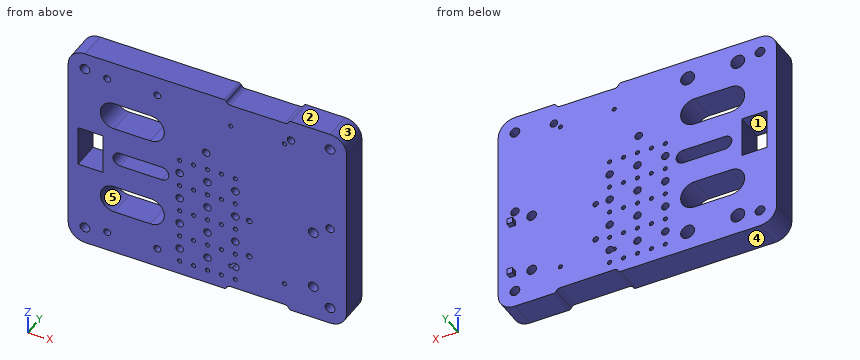
```python
from build123d import *

# Parameters (mm, degrees)
SKETCH_1_W          = 100
SKETCH_1_H          = 75
SKETCH_1_R          = 1.75
SKETCH_1_R_2        = 1.25
SKETCH_1_R_3        = 0.75
SKETCH_1_R_4        = 1.5
SKETCH_1_W_2        = 9
SKETCH_1_H_2        = 14.5
EXTRUDE_1_DEPTH     = 10
FILLET_5_R          = 6
CUT_EXTRUDE_1_REACH = 12
SKETCH_2_R          = 1.35
SKETCH_2_R_2        = 1.75
SKETCH_2_R_3        = 1
SKETCH_3_R          = 2.5
CUT_EXTRUDE_2_DEPTH = 7
SKETCH_4_W          = 2
SKETCH_4_H          = 2
EXTRUDE_2_DEPTH     = 2
CUT_EXTRUDE_3_DEPTH = 36.8
FILLET_6_R          = 1
SKETCH_6_R          = 1.35
SKETCH_6_R_2        = 0.75
CUT_EXTRUDE_4_DEPTH = 36.8


with BuildPart() as part:
    # Эскиз1 → Бобышка-Вытянуть1 (new body)
    with BuildSketch(Plane(origin=(0, 0, 0), x_dir=(1, 0, 0), z_dir=(0, 1, 0))):
        with Locations((50, 37.5)):
            Rectangle(SKETCH_1_W, SKETCH_1_H)
        with Locations((6, 69)):
            Circle(SKETCH_1_R, mode=Mode.SUBTRACT)
        with Locations((94, 69)):
            Circle(SKETCH_1_R, mode=Mode.SUBTRACT)
        with Locations((94, 6)):
            Circle(SKETCH_1_R, mode=Mode.SUBTRACT)
        with Locations((6, 6)):
            Circle(SKETCH_1_R, mode=Mode.SUBTRACT)
        with Locations((14, 68)):
            Circle(SKETCH_1_R_2, mode=Mode.SUBTRACT)
        with Locations((32, 68)):
            Circle(SKETCH_1_R_2, mode=Mode.SUBTRACT)
        with Locations((32, 7)):
            Circle(SKETCH_1_R_2, mode=Mode.SUBTRACT)
        with Locations((14, 7)):
            Circle(SKETCH_1_R_2, mode=Mode.SUBTRACT)
        with Locations((58.35, 65.3)):
            Circle(SKETCH_1_R_3, mode=Mode.SUBTRACT)
        with Locations((77.65, 65.3)):
            Circle(SKETCH_1_R_3, mode=Mode.SUBTRACT)
        with Locations((77.65, 9.7)):
            Circle(SKETCH_1_R_3, mode=Mode.SUBTRACT)
        with Locations((58.35, 9.7)):
            Circle(SKETCH_1_R_3, mode=Mode.SUBTRACT)
        with Locations((94, 37.5)):
            Circle(SKETCH_1_R_4, mode=Mode.SUBTRACT)
        with BuildLine():
            Line((16.5, 59), (29.5, 59))
            ThreePointArc((29.5, 59), (34.5, 54), (29.5, 49))
            Line((29.5, 49), (16.5, 49))
            ThreePointArc((16.5, 49), (11.5, 54), (16.5, 59))
        make_face(mode=Mode.SUBTRACT)
        with BuildLine():
            Line((16.5, 16), (29.5, 16))
            ThreePointArc((29.5, 16), (34.5, 21), (29.5, 26))
            Line((29.5, 26), (16.5, 26))
            ThreePointArc((16.5, 26), (11.5, 21), (16.5, 16))
        make_face(mode=Mode.SUBTRACT)
        with Locations((8, 37.5)):
            Rectangle(SKETCH_1_W_2, SKETCH_1_H_2, mode=Mode.SUBTRACT)
    extrude(amount=EXTRUDE_1_DEPTH)

    # Скругление5
    fillet_5_edges = [part.edges().sort_by_distance(p)[0] for p in [
        (0, 5, -75),
        (100, 5, -75),
        (100, 5, 0),
        (0, 5, 0),
    ]]
    fillet(fillet_5_edges, radius=FILLET_5_R)

    # Эскиз2 → Вырез-Вытянуть1 (cut, up to next)
    with BuildSketch(Plane.XZ, mode=Mode.PRIVATE) as cut_extrude_1_sk1:
        with Locations((80, -7.5)):
            Circle(SKETCH_2_R)
    cut_extrude_1_tool1 = extrude(cut_extrude_1_sk1.sketch, amount=-CUT_EXTRUDE_1_REACH, mode=Mode.PRIVATE) & part.part
    add(cut_extrude_1_tool1.solids().sort_by_distance((80, 0, -7.5))[0], mode=Mode.SUBTRACT)
    # Эскиз2 → Вырез-Вытянуть1 (cut, up to next)
    with BuildSketch(Plane.XZ, mode=Mode.PRIVATE) as cut_extrude_1_sk2:
        with Locations((88, -62.75)):
            Circle(SKETCH_2_R_2)
    cut_extrude_1_tool2 = extrude(cut_extrude_1_sk2.sketch, amount=-CUT_EXTRUDE_1_REACH, mode=Mode.PRIVATE) & part.part
    add(cut_extrude_1_tool2.solids().sort_by_distance((88, 0, -62.75))[0], mode=Mode.SUBTRACT)
    # Эскиз2 → Вырез-Вытянуть1 (cut, up to next)
    with BuildSketch(Plane.XZ, mode=Mode.PRIVATE) as cut_extrude_1_sk3:
        with Locations((88, -41.25)):
            Circle(SKETCH_2_R_2)
    cut_extrude_1_tool3 = extrude(cut_extrude_1_sk3.sketch, amount=-CUT_EXTRUDE_1_REACH, mode=Mode.PRIVATE) & part.part
    add(cut_extrude_1_tool3.solids().sort_by_distance((88, 0, -41.25))[0], mode=Mode.SUBTRACT)
    # Эскиз2 → Вырез-Вытянуть1 (cut, up to next)
    with BuildSketch(Plane.XZ, mode=Mode.PRIVATE) as cut_extrude_1_sk4:
        with Locations((49.550909155, -23.473456754)):
            Circle(SKETCH_2_R)
    cut_extrude_1_tool4 = extrude(cut_extrude_1_sk4.sketch, amount=-CUT_EXTRUDE_1_REACH, mode=Mode.PRIVATE) & part.part
    add(cut_extrude_1_tool4.solids().sort_by_distance((49.550909, 0, -23.473457))[0], mode=Mode.SUBTRACT)
    # Эскиз2 → Вырез-Вытянуть1 (cut, up to next)
    with BuildSketch(Plane.XZ, mode=Mode.PRIVATE) as cut_extrude_1_sk5:
        with Locations((65, -59)):
            Circle(SKETCH_2_R_3)
    cut_extrude_1_tool5 = extrude(cut_extrude_1_sk5.sketch, amount=-CUT_EXTRUDE_1_REACH, mode=Mode.PRIVATE) & part.part
    add(cut_extrude_1_tool5.solids().sort_by_distance((65, 0, -59))[0], mode=Mode.SUBTRACT)
    # Эскиз2 → Вырез-Вытянуть1 (cut, up to next)
    with BuildSketch(Plane.XZ, mode=Mode.PRIVATE) as cut_extrude_1_sk6:
        with Locations((65, -45)):
            Circle(SKETCH_2_R_3)
    cut_extrude_1_tool6 = extrude(cut_extrude_1_sk6.sketch, amount=-CUT_EXTRUDE_1_REACH, mode=Mode.PRIVATE) & part.part
    add(cut_extrude_1_tool6.solids().sort_by_distance((65, 0, -45))[0], mode=Mode.SUBTRACT)
    # Эскиз2 → Вырез-Вытянуть1 (cut, up to next)
    with BuildSketch(Plane.XZ, mode=Mode.PRIVATE) as cut_extrude_1_sk7:
        with BuildLine():
            Line((18.612528652, -35), (33.612528652, -35))
            ThreePointArc((33.612528652, -35), (36.112528652, -37.5), (33.612528652, -40))
            Line((33.612528652, -40), (18.612528652, -40))
            ThreePointArc((18.612528652, -40), (16.112528652, -37.5), (18.612528652, -35))
        make_face()
    cut_extrude_1_tool7 = extrude(cut_extrude_1_sk7.sketch, amount=-CUT_EXTRUDE_1_REACH, mode=Mode.PRIVATE) & part.part
    add(cut_extrude_1_tool7.solids().sort_by_distance((26.112529, 0, -37.5))[0], mode=Mode.SUBTRACT)

    # Эскиз3 → Вырез-Вытянуть2 (cut)
    with BuildSketch(Plane(origin=(0, 10, 0), x_dir=(1, 0, 0), z_dir=(0, 1, 0))):
        with Locations((14, 68)):
            Circle(SKETCH_3_R)
        with Locations((32, 68)):
            Circle(SKETCH_3_R)
        with Locations((14, 7)):
            Circle(SKETCH_3_R)
        with Locations((32, 7)):
            Circle(SKETCH_3_R)
    extrude(amount=-CUT_EXTRUDE_2_DEPTH, mode=Mode.SUBTRACT)

    # Эскиз4 → Бобышка-Вытянуть2 (add)
    with BuildSketch(Plane(origin=(0, 10, 0), x_dir=(1, 0, 0), z_dir=(0, 1, 0))):
        with Locations((94.855745834, 42)):
            Rectangle(SKETCH_4_W, SKETCH_4_H)
        with Locations((94.855745834, 62)):
            Rectangle(SKETCH_4_W, SKETCH_4_H)
    extrude(amount=EXTRUDE_2_DEPTH)

    # Эскиз5 → Вырез-Вытянуть3 (cut)
    with BuildSketch(Plane(origin=(0, 10, 0), x_dir=(1, 0, 0), z_dir=(0, 1, 0))):
        with BuildLine():
            Line((58.204642338, 1.499992816), (77.804642338, 1.439332644))
            ThreePointArc((77.804642338, 1.439332644), (79.299992816, -0.06530251), (77.795357662, -1.560652988))
            Line((77.795357662, -1.560652988), (58.195357662, -1.499992816))
            ThreePointArc((58.195357662, -1.499992816), (56.700007184, 0.004642338), (58.204642338, 1.499992816))
        make_face()
        with BuildLine():
            Line((58.204642338, 73.500007184), (77.804642338, 73.560667356))
            ThreePointArc((77.804642338, 73.560667356), (79.299992816, 75.06530251), (77.795357662, 76.560652988))
            Line((77.795357662, 76.560652988), (58.195357662, 76.499992816))
            ThreePointArc((58.195357662, 76.499992816), (56.700007184, 74.995357662), (58.204642338, 73.500007184))
        make_face()
    extrude(amount=-CUT_EXTRUDE_3_DEPTH, mode=Mode.SUBTRACT)

    # Скругление6
    fillet_6_edges = [part.edges().sort_by_distance(p)[0] for p in [
        (79.298772946, 5, -75),
        (56.7, 5, -75),
        (79.298772946, 5, 0),
        (56.7, 5, 0),
    ]]
    fillet(fillet_6_edges, radius=FILLET_6_R)

    # Эскиз6 → Вырез-Вытянуть4 (cut)
    with BuildSketch(Plane(origin=(0, 10, 0), x_dir=(1, 0, 0), z_dir=(0, 1, 0))):
        with Locations((40, 65)):
            Circle(SKETCH_6_R)
        with Locations((50, 65)):
            Circle(SKETCH_6_R)
        with Locations((60, 65)):
            Circle(SKETCH_6_R)
        with Locations((50, 55)):
            Circle(SKETCH_6_R)
        with Locations((60, 55)):
            Circle(SKETCH_6_R)
        with Locations((50, 45)):
            Circle(SKETCH_6_R)
        with Locations((60, 45)):
            Circle(SKETCH_6_R)
        with Locations((50, 35)):
            Circle(SKETCH_6_R)
        with Locations((60, 35)):
            Circle(SKETCH_6_R)
        with Locations((40, 55)):
            Circle(SKETCH_6_R)
        with Locations((40, 45)):
            Circle(SKETCH_6_R)
        with Locations((40, 35)):
            Circle(SKETCH_6_R)
        with Locations((40, 70)):
            Circle(SKETCH_6_R_2)
        with Locations((45, 70)):
            Circle(SKETCH_6_R_2)
        with Locations((50, 70)):
            Circle(SKETCH_6_R_2)
        with Locations((55, 70)):
            Circle(SKETCH_6_R_2)
        with Locations((60, 70)):
            Circle(SKETCH_6_R_2)
        with Locations((45, 60)):
            Circle(SKETCH_6_R_2)
        with Locations((50, 60)):
            Circle(SKETCH_6_R_2)
        with Locations((55, 60)):
            Circle(SKETCH_6_R_2)
        with Locations((60, 60)):
            Circle(SKETCH_6_R_2)
        with Locations((45, 50)):
            Circle(SKETCH_6_R_2)
        with Locations((50, 50)):
            Circle(SKETCH_6_R_2)
        with Locations((55, 50)):
            Circle(SKETCH_6_R_2)
        with Locations((60, 50)):
            Circle(SKETCH_6_R_2)
        with Locations((45, 40)):
            Circle(SKETCH_6_R_2)
        with Locations((50, 40)):
            Circle(SKETCH_6_R_2)
        with Locations((55, 40)):
            Circle(SKETCH_6_R_2)
        with Locations((60, 40)):
            Circle(SKETCH_6_R_2)
        with Locations((45, 30)):
            Circle(SKETCH_6_R_2)
        with Locations((50, 30)):
            Circle(SKETCH_6_R_2)
        with Locations((55, 30)):
            Circle(SKETCH_6_R_2)
        with Locations((60, 30)):
            Circle(SKETCH_6_R_2)
        with Locations((40, 60)):
            Circle(SKETCH_6_R_2)
        with Locations((40, 50)):
            Circle(SKETCH_6_R_2)
        with Locations((40, 40)):
            Circle(SKETCH_6_R_2)
        with Locations((40, 30)):
            Circle(SKETCH_6_R_2)
    extrude(amount=-CUT_EXTRUDE_4_DEPTH, mode=Mode.SUBTRACT)


solid = part.part
```
Check sheet for the modelled part. Datum: model origin and axes. Units: mm. Face numbers are marked on the shaded views. A direction names the side the tool comes from. Give positions to 0.01 mm unless a question says otherwise; leave off trailing zeros. Loops run counter-clockwise (first coordinate to the right, second up) from the corner with the lowest first, then second, coordinate; pieces in that order, holes last. Notation, with made-up numbers: (-18.75, 23) - (31.25, 23) arc R33 ccw to (31.25, 53) - close; hole circle Ø8 at (47.5, -19.75). An arc over 180 degrees is marked (long way). One line per question, with ' | ' between items. Start each with the question number.
1. Cross-section at D-D, the plane x = 69.5. Enter the section's corners in (y, z).
2. Material ranges on line 1 along Z through (x, y) = (94, 3.5); line 2 along Z through (x, y) = (6, 5); line 3 along Z through (x, y) = (45, 3.5), recorded low to high. Write a range as [from, to].
3. Gauge pin test, flat ends, axial feed: pin 1 Ø6.5 at (x, z) = (14, -68) entering from +Y; pin 2 Ø1.7 at (x, z) = (45, -50) entering from -Y; pin 3 Ø1 at (x, y) = (95, 11.5) entering from -Z; pin 4 Ø3 at (x, z) = (32, -68) entering from +Y. Record the tip position at first contact, or that the pin passes through.
4. Cross-section at C-C, the plane y = 1.25. Give the number of separate pieces and of enclosed holes in the cut face, plus the area to 3 significant figures.
5. Set-up check for the marked faces 4 and 5: record each of +Z, -Z, +X, -X, +Y, -Y from which the full face is reachable in a straight line by a thin tool's end or side.
6. Draft check along X on the marked faces 1, 2 and 3. Enter one of: released by +X, released by -X, zero draft, split by the parting line, or undercut.
7. Cross-section at A-A, the plane x = 24.5. Enter the section's corners in (y, z).
8. Cross-section at B-B, the plane z = -12. Enter the section's corners in (x, y).
Check result:
1) outline: (0, -73.53) - (10, -73.53) - (10, -1.47) - (0, -1.47) - close
2) line 1: z = [-75, -70.75], [-67.25, -39], [-36, -7.75], [-4.25, 0] | line 2: z = [-75, -70.75], [-67.25, -44.75], [-30.25, -7.75], [-4.25, 0] | line 3: z = [-75, -70.75], [-69.25, -60.75], [-59.25, -50.75], [-49.25, -40.75], [-39.25, -30.75], [-29.25, 0]
3) pin 1: stops at y = 10 | pin 2: stops at y = 0 | pin 3: stops at z = -63 | pin 4: stops at y = 3
4) separate pieces: 1 | enclosed holes: 59 | area: 6,540 mm2
5) face 4: -Z, +X, -X, +Y, -Y | face 5: +Y, -Y
6) face 1: undercut | face 2: zero draft | face 3: released by +X
7) outline: (0, -75) - (10, -75) - (10, -59) - (0, -59) - close; (0, -49) - (10, -49) - (10, -40) - (0, -40) - close; (0, -35) - (10, -35) - (10, -26) - (0, -26) - close; (0, -16) - (10, -16) - (10, 0) - (0, 0) - close
8) outline: (0, 0) - (100, 0) - (100, 10) - (0, 10) - close
